from build123d import *

# Parameters (mm, degrees)
F0_W      = 80
F0_H      = 50
F1_DEPTH  = 25
F3_DEPTH  = 25
F4_W      = 25
F4_H      = 10
F5_DEPTH  = 25
F7_D      = 4.4
F7_DEPTH  = 25
F7_TIP    = 1.3218933619
F8_W      = 30
F8_H      = 3
F9_DEPTH  = 25
F11_DEPTH = 25
F13_D     = 3.2
F13_DEPTH = 15
F13_TIP   = 0.9613769904


with BuildPart() as f1:
    # F0 (on Front) → F1 (new body)
    with BuildSketch(Plane.XZ):
        Rectangle(F0_W, F0_H)
    extrude(amount=F1_DEPTH)

    # F2 (on face) → F3 (cut)
    with BuildSketch(Plane.XZ.offset(25)):
        Polygon((-35, -25), (-40, -20), (-40, -25), align=None)
        Polygon((-40, 20), (-35, 25), (-40, 25), align=None)
    extrude(amount=-F3_DEPTH, mode=Mode.SUBTRACT)

    # F4 (on face) → F5 (cut)
    with BuildSketch(Plane.XZ.offset(25)):
        with Locations((-27.5, 0)):
            Rectangle(F4_W, F4_H)
    extrude(amount=-F5_DEPTH, mode=Mode.SUBTRACT)

    # F7
    with Locations(Plane(origin=(-15, 0, 0), x_dir=(0, -1, 0), z_dir=(-1, 0, 0))):
        with Locations((12.5, 0)):
            Hole(F7_D / 2, depth=F7_DEPTH)
            with Locations((0, 0, -(F7_DEPTH + F7_TIP / 2))):  # 118° drill point
                Cone(0, F7_D / 2, F7_TIP, mode=Mode.SUBTRACT)

    # F8 (on face) → F9 (cut)
    with BuildSketch(Plane.XZ.offset(25)):
        with Locations((25, -23.5)):
            Rectangle(F8_W, F8_H)
        with Locations((25, 23.5)):
            Rectangle(F8_W, F8_H)
    extrude(amount=-F9_DEPTH, mode=Mode.SUBTRACT)

    # F10 (on face) → F11 (cut)
    with BuildSketch(Plane.XZ.offset(25)):
        Polygon((34.5029532909, -16.7983844876), (40, -22), (40, 22), (37.8786325455, 22), (35.2007597685, 18.9214255661), (37.6393385231, 16.1444209516), (37.6393385231, 14.2828542739), (38.1201058626, 10.1062655449), (36.3511256874, 7.2423182428), (38.3169800043, 4.507265985), (37.0589233935, 1.4836080372), (37.0589233935, -2.0621158183), (35.0656695664, -5.7143010199), (38.1139032543, -8.7043344975), (35.661585629, -11.3277509809), (36.5576688207, -14.626969239), align=None)
    extrude(amount=-F11_DEPTH, mode=Mode.SUBTRACT)

    # F13
    with Locations(Plane.XY.offset(22)):
        with Locations((23.9393162727, -12.5)):
            Hole(F13_D / 2, depth=F13_DEPTH)
            with Locations((0, 0, -(F13_DEPTH + F13_TIP / 2))):  # 118° drill point
                Cone(0, F13_D / 2, F13_TIP, mode=Mode.SUBTRACT)


solid = f1.part
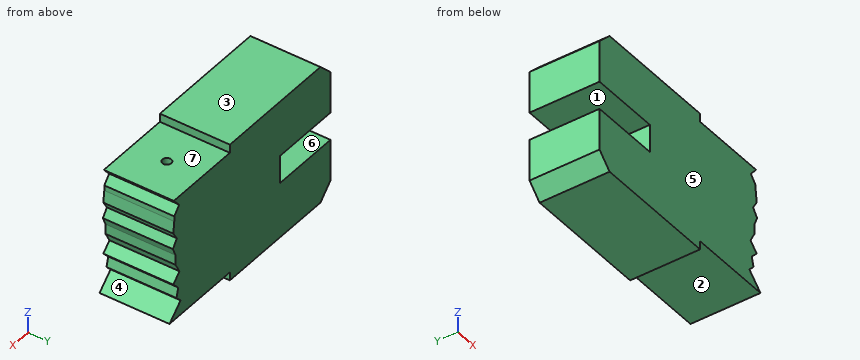
Verification items for the finished model (mm, model axes). Face numbers are marked on the shaded views. A direction names the side the tool comes from. Coordinates: 2 decimals unless noted, no trailing zeros. Loops run counter-clockwise (first coordinate to the right, second up) from the corner with the lowest first, then second, coordinate; pieces in that order, holes last. Notation, with made-up numbers: (34, -3) -> (89, -3) arc R15 ccw to (89, 4) -> close; hole circle Ø5 at (67, 67.5). An arc over 180 degrees is marked (long way). Answer as CSV lines item,"result".
1) Depth check by flat-ended pin: pin 1 (12.5 mm diameter, centred on x = 19.5, y = -11, fed in from -Z); pin 2 (2.5 mm diameter, centred on y = -8, z = -24, fed in from +X); pin 3 (2 mm diameter, centred on y = -13, z = 15, fed in from +X). Enter the tip coordinate at first touch or a pass-through.
Found:
pin 1,"stops at z = -22"
pin 2,"stops at x = 10"
pin 3,"stops at x = 37.67"
2) Cross-section at B-B, the plane y = -20.5. Record the cut outline in (x, z).
Found:
outline,"(-40, -20) -> (-35, -25) -> (10, -25) -> (10, -22) -> (40, -22) -> (34.5, -16.8) -> (36.56, -14.63) -> (35.66, -11.33) -> (38.11, -8.7) -> (35.07, -5.71) -> (37.06, -2.06) -> (37.06, 1.48) -> (38.32, 4.51) -> (36.35, 7.24) -> (38.12, 10.11) -> (37.64, 14.28) -> (37.64, 16.14) -> (35.2, 18.92) -> (37.88, 22) -> (10, 22) -> (10, 25) -> (-35, 25) -> (-40, 20) -> (-40, 5) -> (-15, 5) -> (-15, -5) -> (-40, -5) -> close"
3) Cross-section at A-A, the plane x = -26. Record the cut outline in (y, z).
Found:
outline,"(-25, -25) -> (0, -25) -> (0, -5) -> (-25, -5) -> close; (-25, 5) -> (0, 5) -> (0, 25) -> (-25, 25) -> close"
4) Thickness scan on L1, parallel to Y at x = -7.75, z = 0; L2, parallel to Z at x = -28.5, y = -7; L3, parallel to Z at x = 1.5, y = -12.25. Record the ranges inside material, lowest first. Write a range as from..to.
Found:
L1,"y = -25..-14.7, -10.3..0"
L2,"z = -25..-5, 5..25"
L3,"z = -25..-2.19, 2.19..25"
5) Tool access check on the marked faces 1, 2, 3 and 4. Record the directions out of +Z, -Z, +X, -X, +Y, -Y that give a thin tool (end or side, any length) a straight path to the whole face; none if there is none.
Found:
face 1,"-X, +Y, -Y"
face 2,"-Z, +X, +Y, -Y"
face 3,"+Z, +X, -X, +Y, -Y"
face 4,"+X, +Y, -Y"
6) Release check for a two-part mould opening along Z. For the marked faces 5, 6 and 7 record: +Z half, -Z half, draft (parallel to the pull), parting line (faces both ways), or undercut.
Found:
face 5,"draft"
face 6,"undercut"
face 7,"+Z half"
7) Cross-section at C-C, the plane x = 33. Record the cut outline in (y, z).
Found:
outline,"(-25, -22) -> (0, -22) -> (0, 22) -> (-25, 22) -> close"
8) Cross-section at D-D, the plane z = 13.5. Record the cut outline in (x, y), then the cut area to 3 significant figures.
Found:
outline,"(-40, -25) -> (37.73, -25) -> (37.73, 0) -> (-40, 0) -> close; hole circle Ø3.2 at (23.94, -12.5)"
area,"1,940 mm2"
